Here's the drawing with two shaded views (mm, measured from the low corner). I have some questions. Round coordinates to 2 decimals unless told otherwise and drop trailing zeros. Use a Markdown table: item, result.
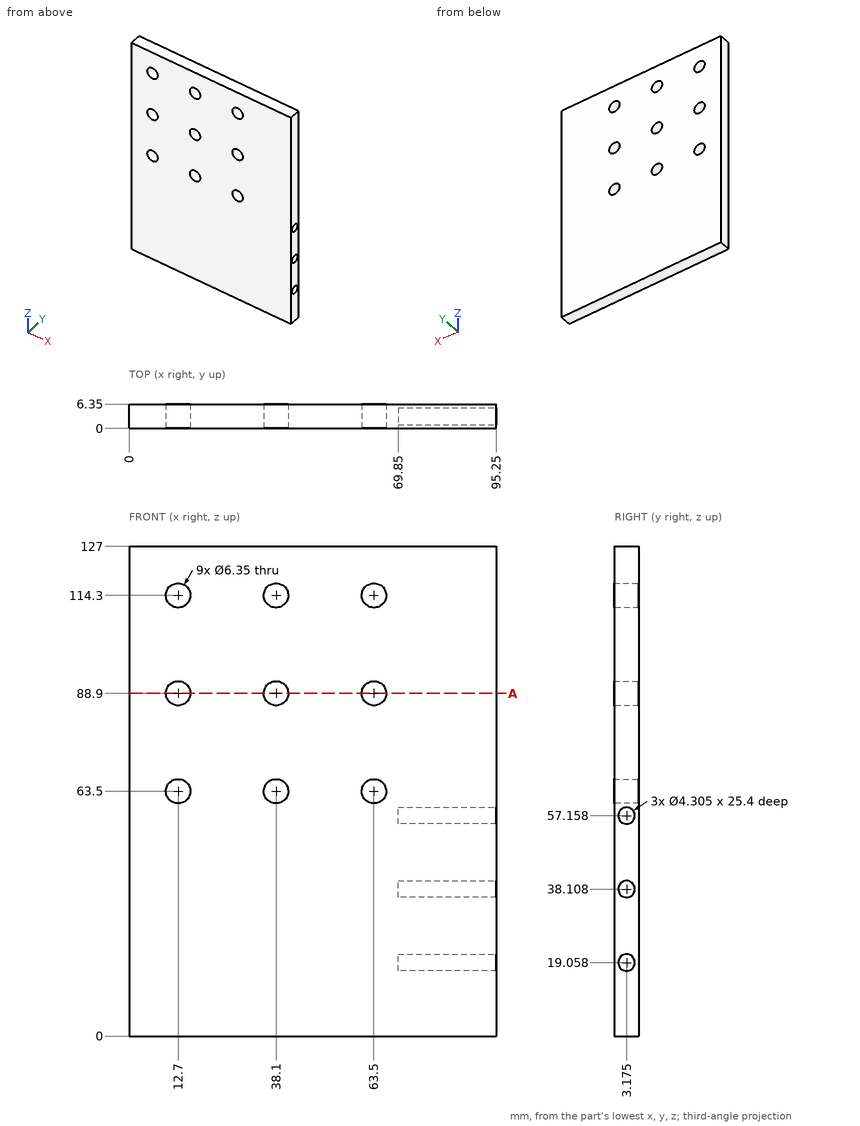
1. I need wall thicknesses on line 1 (Z direction, x = 65, y = 4.25). Which ranges of the line are inside material? Lowest first, please.
Answer sheet:
| item | result |
|---|---|
| line 1 | z = 0 to 60.7, 66.3 to 86.1, 91.7 to 111.5, 117.1 to 127 |
2. I want a section at A-A (z = 88.9). State how many separate pieces and enclosed holes the cut face has, plus the area to 3 significant figures.
Answer sheet:
| item | result |
|---|---|
| separate pieces | 4 |
| enclosed holes | 0 |
| area | 484 mm² |
3. Will these pins go through, and if not, where does the flat tip stop? pin 1 Ø5 at (x, z) = (12.7, 88.9) entering from +Y; pin 2 Ø12 at (x, z) = (25, 14.5) entering from -Y; pin 3 Ø1.3 at (y, z) = (3, 57) entering from +X.
Answer sheet:
| item | result |
|---|---|
| pin 1 | passes through |
| pin 2 | stops at y = 0 |
| pin 3 | stops at x = 69.85 |
